Design review of the part built by this model. Coordinates are the model's own, in mm. A direction names the side the tool comes from. Give positions to 0.01 mm unless a question says otherwise; leave off trailing zeros. Loops run counter-clockwise (first coordinate to the right, second up) from the corner with the lowest first, then second, coordinate; pieces in that order, holes last.
from build123d import *

# Parameters (mm, degrees)
SKETCH1_W                 = 54
SKETCH1_H                 = 48
SKETCH1_R                 = 2
BOSS_EXTRUDE1_DEPTH       = 5
SKETCH2_W                 = 10
SKETCH2_H                 = 48
BOSS_EXTRUDE2_DEPTH       = 72.5
SKETCH3_W                 = 48
SKETCH3_H                 = 10
BOSS_EXTRUDE3_DEPTH       = 30
FILLET1_R                 = 10
CHAMFER1_SIZE             = 11
F_1_0MM_START             = -72.5
F_1_0MM_DOWEL_SLOT1_DEPTH = 10
FILLET2_R                 = 10


# Read off the part's stored shape, not the designer's step: Ø1.0mm Dowel Slot1
with BuildPart() as part:
    # Sketch1 → Boss-Extrude1 (new body)
    with BuildSketch(Plane(origin=(0, 0, 0), x_dir=(1, 0, 0), z_dir=(0, 1, 0))):
        with Locations((3, 0)):
            Rectangle(SKETCH1_W, SKETCH1_H)
        with Locations(Location((0.133743503, 17.499488926, 0), (0, 0, 270))):
            Circle(SKETCH1_R, mode=Mode.SUBTRACT)
        with Locations(Location((0, -17.5, 0), (0, 0, 270))):
            Circle(SKETCH1_R, mode=Mode.SUBTRACT)
        with BuildLine():
            Line((19.068905623, 9), (11.068905623, 9))
            ThreePointArc((11.068905623, 9), (-14, 0), (11.068905623, -9))
            Line((11.068905623, -9), (19.068905623, -9))
            Line((19.068905623, -9), (19.068905623, 9))
        make_face(mode=Mode.SUBTRACT)
    extrude(amount=BOSS_EXTRUDE1_DEPTH)

    # Sketch2 → Boss-Extrude2 (add)
    with BuildSketch(Plane.XZ):
        with Locations((25, 0)):
            Rectangle(SKETCH2_W, SKETCH2_H)
    extrude(amount=BOSS_EXTRUDE2_DEPTH)

    # Sketch3 → Boss-Extrude3 (add)
    with BuildSketch(Plane(origin=(30, 0, 0), x_dir=(0, 0, -1), z_dir=(1, 0, 0))):
        with Locations((0, -67.5)):
            Rectangle(SKETCH3_W, SKETCH3_H)
    extrude(amount=BOSS_EXTRUDE3_DEPTH)

    # Fillet1
    fillet1_edges = [part.edges().sort_by_distance(p)[0] for p in [
        (-24, 2.5, -24),
        (-24, 2.5, 24),
    ]]
    fillet(fillet1_edges, radius=FILLET1_R)

    # Chamfer1
    # the kernel refuses this chamfer: 11 mm, written as the material it adds along each edge
    with BuildSketch(Plane(origin=(20, 0, 24), x_dir=(-0.9996219169112968, 0.027495876610586372, 0), z_dir=(0, 0, -1))) as chamfer1_piece_1_section:
        Polygon((CHAMFER1_SIZE * 0.999621916911, -CHAMFER1_SIZE * 0.0274958766106), (-CHAMFER1_SIZE * 0.0274958766106, -CHAMFER1_SIZE * 0.999621916911), (0, 0), align=None)
    chamfer1_piece_1 = extrude(amount=48, mode=Mode.PRIVATE)
    chamfer1_piece_1 = split(chamfer1_piece_1, bisect_by=Plane(origin=(15.585058089, -3.181005548, 9), z_dir=(0, 0, 1)), keep=Keep.TOP, mode=Mode.PRIVATE)
    chamfer1_piece_1 = chamfer1_piece_1 - Plane(origin=(0.15, -3.181005548, 0), x_dir=(0.7716541076196256, 0, -0.6360424028268551), z_dir=(0, -1, 0)) * Cylinder(14.15, 140, mode=Mode.PRIVATE)
    chamfer1_piece_1 = split(chamfer1_piece_1, bisect_by=Plane(origin=(19.068905623, -3.181005548, 16.524598141), z_dir=(-1, 0, 0)), keep=Keep.TOP, mode=Mode.PRIVATE)
    add(chamfer1_piece_1)
    with BuildSketch(Plane(origin=(20, 0, 24), x_dir=(-0.9996219169112968, 0.027495876610586372, 0), z_dir=(0, 0, -1))) as chamfer1_piece_2_section:
        Polygon((CHAMFER1_SIZE * 0.999621916911, -CHAMFER1_SIZE * 0.0274958766106), (-CHAMFER1_SIZE * 0.0274958766106, -CHAMFER1_SIZE * 0.999621916911), (0, 0), align=None)
    chamfer1_piece_2 = extrude(amount=48, mode=Mode.PRIVATE)
    chamfer1_piece_2 = split(chamfer1_piece_2, bisect_by=Plane(origin=(19.684713813, -5.503387728, 9), z_dir=(0, 0, 1)), keep=Keep.TOP, mode=Mode.PRIVATE)
    chamfer1_piece_2 = split(chamfer1_piece_2, bisect_by=Plane(origin=(19.068905623, -5.503387728, 16.5), z_dir=(1, 0, 0)), keep=Keep.TOP, mode=Mode.PRIVATE)
    add(chamfer1_piece_2)
    with BuildSketch(Plane(origin=(20, 0, 24), x_dir=(-0.9996219169112968, 0.027495876610586372, 0), z_dir=(0, 0, -1))) as chamfer1_piece_3_section:
        Polygon((CHAMFER1_SIZE * 0.999621916911, -CHAMFER1_SIZE * 0.0274958766106), (-CHAMFER1_SIZE * 0.0274958766106, -CHAMFER1_SIZE * 0.999621916911), (0, 0), align=None)
    chamfer1_piece_3 = extrude(amount=48, mode=Mode.PRIVATE)
    chamfer1_piece_3 = split(chamfer1_piece_3, bisect_by=Plane(origin=(19.684713813, -5.503387728, 9), z_dir=(0, 0, -1)), keep=Keep.TOP, mode=Mode.PRIVATE)
    chamfer1_piece_3 = split(chamfer1_piece_3, bisect_by=Plane(origin=(19.068905623, -5.503387728, 0), z_dir=(1, 0, 0)), keep=Keep.TOP, mode=Mode.PRIVATE)
    chamfer1_piece_3 = split(chamfer1_piece_3, bisect_by=Plane(origin=(19.684713813, -5.503387728, -9), z_dir=(0, 0, 1)), keep=Keep.TOP, mode=Mode.PRIVATE)
    add(chamfer1_piece_3)
    with BuildSketch(Plane(origin=(20, 0, 24), x_dir=(-0.9996219169112968, 0.027495876610586372, 0), z_dir=(0, 0, -1))) as chamfer1_piece_4_section:
        Polygon((CHAMFER1_SIZE * 0.999621916911, -CHAMFER1_SIZE * 0.0274958766106), (-CHAMFER1_SIZE * 0.0274958766106, -CHAMFER1_SIZE * 0.999621916911), (0, 0), align=None)
    chamfer1_piece_4 = extrude(amount=48, mode=Mode.PRIVATE)
    chamfer1_piece_4 = chamfer1_piece_4 - Plane(origin=(0.15, -3.181005547, 0), x_dir=(0.7716541076196256, 0, -0.6360424028268551), z_dir=(0, -1, 0)) * Cylinder(14.15, 140, mode=Mode.PRIVATE)
    chamfer1_piece_4 = split(chamfer1_piece_4, bisect_by=Plane(origin=(19.068905623, -3.181005547, -16.524598139), z_dir=(-1, 0, 0)), keep=Keep.TOP, mode=Mode.PRIVATE)
    chamfer1_piece_4 = split(chamfer1_piece_4, bisect_by=Plane(origin=(15.585058087, -3.181005547, -9), z_dir=(0, 0, -1)), keep=Keep.TOP, mode=Mode.PRIVATE)
    add(chamfer1_piece_4)
    with BuildSketch(Plane(origin=(20, 0, 24), x_dir=(-0.9996219169112968, 0.027495876610586372, 0), z_dir=(0, 0, -1))) as chamfer1_piece_5_section:
        Polygon((CHAMFER1_SIZE * 0.999621916911, -CHAMFER1_SIZE * 0.0274958766106), (-CHAMFER1_SIZE * 0.0274958766106, -CHAMFER1_SIZE * 0.999621916911), (0, 0), align=None)
    chamfer1_piece_5 = extrude(amount=48, mode=Mode.PRIVATE)
    chamfer1_piece_5 = split(chamfer1_piece_5, bisect_by=Plane(origin=(19.068905623, -5.503387728, -16.5), z_dir=(1, 0, 0)), keep=Keep.TOP, mode=Mode.PRIVATE)
    chamfer1_piece_5 = split(chamfer1_piece_5, bisect_by=Plane(origin=(19.684713813, -5.503387728, -9), z_dir=(0, 0, -1)), keep=Keep.TOP, mode=Mode.PRIVATE)
    add(chamfer1_piece_5)
    with BuildSketch(Plane(origin=(30, -62.5, -24), x_dir=(-0.02749587661058594, 0.9996219169112968, 0), z_dir=(0, 0, 1))) as chamfer1_piece_6:
        Polygon((CHAMFER1_SIZE * 0.999621916911, -CHAMFER1_SIZE * 0.0274958766106), (-CHAMFER1_SIZE * 0.0274958766106, -CHAMFER1_SIZE * 0.999621916911), (0, 0), align=None)
    extrude(amount=48)

    # Ø1.0mm Dowel Slot1 outline → Ø1.0mm Dowel Slot1 (cut)
    with BuildSketch(Plane(origin=(0, 0, 0), x_dir=(1, 0, 0), z_dir=(0, 1, 0)).offset(F_1_0MM_START)):
        with BuildLine():
            Line((48, 9.25), (53, 9.25))
            ThreePointArc((53, 9.25), (55.75, 12), (53, 14.75))
            Line((53, 14.75), (48, 14.75))
            ThreePointArc((48, 14.75), (45.25, 12), (48, 9.25))
        make_face()
        with BuildLine():
            Line((48, -14.75), (53, -14.75))
            ThreePointArc((53, -14.75), (55.75, -12), (53, -9.25))
            Line((53, -9.25), (48, -9.25))
            ThreePointArc((48, -9.25), (45.25, -12), (48, -14.75))
        make_face()
    extrude(amount=F_1_0MM_DOWEL_SLOT1_DEPTH, mode=Mode.SUBTRACT)

    # Fillet2
    fillet2_edges = [part.edges().sort_by_distance(p)[0] for p in [
        (60, -67.5, 24),
        (60, -67.5, -24),
    ]]
    fillet(fillet2_edges, radius=FILLET2_R)


solid = part.part
Q1. Take a section at C-C (z = 16.5). Give the boundary of the cut face in (x, y).
Results:
outline: (-23.68, 0) - (-1.73, 0) - (-1.73, 5) - (-23.68, 5) - close; (1.73, 0) - (9, 0) - (20, -11) - (20, -72.5) - (59.68, -72.5) - (59.68, -62.5) - (41, -62.5) - (30, -51.5) - (30, 5) - (1.73, 5) - close
Q2. Take a section at A-A (x = 15.5). Give the boundary of the cut face in (y, z).
Results:
outline: (-6.5, -24) - (5, -24) - (5, -9) - (-6.5, -9) - close; (-6.5, 9) - (5, 9) - (5, 24) - (-6.5, 24) - close
Q3. Draft analysis for pull direction X (two halves, no side actions). For faces 1 (the face through (60, -67, 0)), 2 (the face through (40, -72.5, 0)), 3 (the face through (55.75, -67.57, -11.94)), state which applies: pulls with the +X half, pulls with the -X half, needs draft (parallel to the pull), parting line crosses it, or undercut.
Results:
face 1: pulls with the +X half
face 2: needs draft
face 3: undercut
Q4. Tool access review of faces 4 (the face through (50, -62.5, 0)), 5 (the face through (20, -41, 0)), 6 (the face through (15, -1, 9)): name each direction out of +Z, -Z, +X, -X, +Y, -Y from which nothing blocks a thin tool from reaching the whole face with its end or side.
Results:
face 4: +Z, -Z, +X, +Y
face 5: +Z, -Z, -X, -Y
face 6: +Y, -Y
Q5. Insertion check: pin 1 (1 mm diameter, centred on x = 11.5, y = -3, fed in from -Z); pin 2 (1.5 mm diameter, centred on x = 39, z = -11.5, fed in from +Y); pin 3 (4.5 mm diameter, centred on y = -2.5, z = -3, fed in from -X); pin 4 (24 mm diameter, centred on y = -45, z = 6, fed in from -X). Each pin has a flat end and moves straight along its axis. Give the tip position at first contact, or say it passes through.
Results:
pin 1: stops at z = -24
pin 2: stops at y = -59.75
pin 3: stops at x = 19.07
pin 4: stops at x = 20
Q6. Take a section at B-B (z = 0). Give the boundary of the cut face in (x, y), plus the area to 3 significant figures.
Results:
outline: (-24, 0) - (-14, 0) - (-14, 5) - (-24, 5) - close; (19.07, -10.07) - (20, -11) - (20, -72.5) - (60, -72.5) - (60, -62.5) - (41, -62.5) - (30, -51.5) - (30, 5) - (19.07, 5) - close
area: 1,200 mm2
Q7. Wall thickness on line 1 (X direction, y = 3, z = 0); line 2 (X direction, y = -43, z = -3); line 3 (Y direction, x = 7.5, z = 15): over which ranges is each line inside the solid? List them lowest first.
Results:
line 1: x = -24 to -14, 19.07 to 30
line 2: x = 20 to 30
line 3: y = 0 to 5
Q8. Take a section at D-D (x = -5.5). Give the boundary of the cut face in (y, z), plus the area to 3 significant figures.
Results:
outline: (0, -24) - (5, -24) - (5, -12.97) - (0, -12.97) - close; (0, 12.97) - (5, 12.97) - (5, 24) - (0, 24) - close
area: 110 mm2
